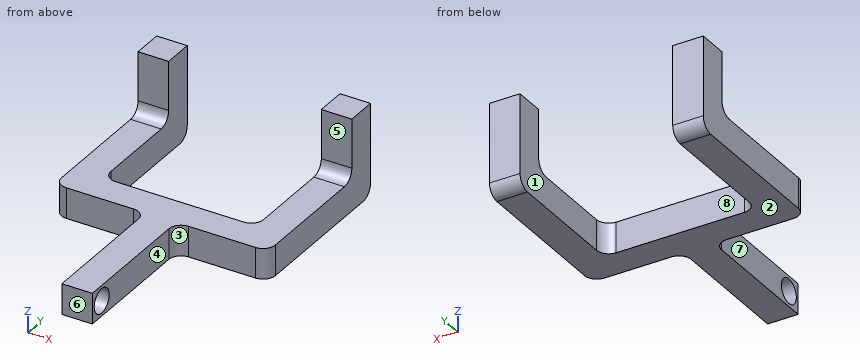
```python
from build123d import *

# Parameters (mm, degrees)
BOSS_EXTRU_1_DEPTH                = 10
ESQUISSE2_W                       = 10
ESQUISSE2_H                       = 10
BOSS_EXTRU_2_DEPTH                = 20
DIAM_TRE_DU_PER_AGE_8_0_8_1_D     = 8
DIAM_TRE_DU_PER_AGE_8_0_8_1_DEPTH = 10
DIAM_TRE_DU_PER_AGE_8_0_8_1_TIP   = 2.403442476
CONG_1_R                          = 4


with BuildPart() as part:
    # Esquisse1 → Boss.-Extru.1 (new body)
    with BuildSketch(Plane.XY):
        Polygon((30, 0), (30, 45), (0, 45), (0, 100), (10, 100), (10, 55), (60, 55), (60, 100), (70, 100), (70, 45), (40, 45), (40, 0), align=None)
    extrude(amount=BOSS_EXTRU_1_DEPTH)

    # Esquisse2 → Boss.-Extru.2 (add)
    with BuildSketch(Plane.XY.offset(10)):
        with Locations((5, 95)):
            Rectangle(ESQUISSE2_W, ESQUISSE2_H)
        with Locations((65, 95)):
            Rectangle(ESQUISSE2_W, ESQUISSE2_H)
    extrude(amount=BOSS_EXTRU_2_DEPTH)

    # Diamètre du perçage Ø8.0 (8)1
    with Locations(Plane.ZY.offset(-30)):
        with Locations((5, 5)):
            Hole(DIAM_TRE_DU_PER_AGE_8_0_8_1_D / 2, depth=DIAM_TRE_DU_PER_AGE_8_0_8_1_DEPTH)
            with Locations((0, 0, -(DIAM_TRE_DU_PER_AGE_8_0_8_1_DEPTH + DIAM_TRE_DU_PER_AGE_8_0_8_1_TIP / 2))):  # 118° drill point
                Cone(0, DIAM_TRE_DU_PER_AGE_8_0_8_1_D / 2, DIAM_TRE_DU_PER_AGE_8_0_8_1_TIP, mode=Mode.SUBTRACT)

    # Congé1
    cong_1_edges = [part.edges().sort_by_distance(p)[0] for p in [
        (5, 100, 0),
        (65, 100, 0),
        (70, 45, 5),
        (40, 45, 5),
        (30, 45, 5),
        (0, 45, 5),
        (10, 55, 5),
        (60, 55, 5),
        (5, 90, 10),
        (65, 90, 10),
    ]]
    fillet(cong_1_edges, radius=CONG_1_R)


solid = part.part
```
CAD build for the part. Positions are in the model's coordinates, mm. Face numbers are marked on the shaded views. A direction names the side the tool comes from. Round coordinates to 2 decimals unless told otherwise and drop trailing zeros. Loops run counter-clockwise (first coordinate to the right, second up) from the corner with the lowest first, then second, coordinate; pieces in that order, holes last. Notation, with made-up numbers: M -20.75,-17.5 L 4.25,-17.5 A24 cw 4.25,-7.5 Z; hole C 17.5,82.25 d1. An arc over 180 degrees is marked long. Use a Markdown table: item, result. Add a question column.
(1) Which spindle directions (+Z, -Z, +X, -X, +Y, -Y) get a long thin tool onto all of the face, cutting with end or side? Do the marked faces 4, 5, 6, 7 and 8. Say none if no direction does.
(2) Pull direction X, two halves, no side cores. Call the marked faces 1, 2 and 3: +X half, -X half, draft (parallel to the pull), parting line (faces both ways), or undercut.
(3) Cut at C-C (z = 12.75). Give the cut face in (x, y), and give its area (3 significant figures).
(4) Cut at A-A (y = 66). Give the cut face in (x, z).
(5) Cut at B-B (x = 34.5). Give the cut face in (y, z).
(6) Cut at D-D (x = 8.5). Give the cut face in (y, z), and give its area (3 significant figures).
(7) Flat gauge pins, fed straight in: pin 1 (5 mm diameter, centred on x = 15.5, z = 7.5, fed in from -Y); pin 2 (8 mm diameter, centred on y = 13.5, z = 6, fed in from -X); pin 3 (11 mm diameter, centred on y = 30, z = 4, fed in from +X); pin 4 (2 mm diameter, centred on y = 61, z = 12, fed in from -X). Where does each tip first touch, or does it go through?
(8) Drill centre lines: line 1 (X direction, y = 91.5, z = 16.75); line 2 (Z direction, x = 37.5, y = 5); line 3 (Y direction, x = 37.75, z = 5). Where is each one in solid material? Low to high.
Geometry says:
| question | item | result |
|---|---|---|
| 1 | face 4 | +Z, -Z, +X, -Y |
| 1 | face 5 | +Z, +X, -X, -Y |
| 1 | face 6 | +Z, -Z, +X, -X, -Y |
| 1 | face 7 | +Z, -Z, -X, -Y |
| 1 | face 8 | +Z, -Z, +Y |
| 2 | face 1 | undercut |
| 2 | face 2 | draft |
| 2 | face 3 | +X half |
| 3 | outline | M 0,89.8 L 10,89.8 L 10,100 L 0,100 Z; M 60,89.8 L 70,89.8 L 70,100 L 60,100 Z |
| 3 | area | 204 mm² |
| 4 | outline | M 0,0 L 10,0 L 10,10 L 0,10 Z; M 60,0 L 70,0 L 70,10 L 60,10 Z |
| 5 | outline | M 0,0 L 55,0 L 55,10 L 0,10 Z; hole C 5,5 d8 |
| 6 | outline | M 45,0 L 96,0 A4 ccw 100,4 L 100,30 L 90,30 L 90,14 A4 cw 86,10 L 45,10 Z |
| 6 | area | 750 mm² |
| 7 | pin 1 | stops at y = 45 |
| 7 | pin 2 | stops at x = 30 |
| 7 | pin 3 | stops at x = 40 |
| 7 | pin 4 | passes through |
| 8 | line 1 | x = 0 to 10, 60 to 70 |
| 8 | line 2 | z = 0 to 1, 9 to 10 |
| 8 | line 3 | y = 0 to 1, 9 to 55 |
